Autodesk Inventor part; units mm, degrees
ref_plane "YZ Plane" through (0, 0, 0) normal (1, 0, 0) x (0, 1, 0)
ref_plane "XZ Plane" through (0, 0, 0) normal (0, 1, 0) x (-1, 0, 0)
ref_plane "XY Plane" through (0, 0, 0) normal (0, 0, 1) x (1, 0, 0)
sketch "Sketch1" plane through (0, 0, 0) normal (0, 0, 1) x (1, 0, 0)
  line L0 (2, 0) -> (8, 0)
  line L1 (10, 2) -> (10, 13)
  line L2 (8, 15) -> (2, 15)
  line L3 (0, 13) -> (0, 2)
  circle A0 centre (5, 7.5) radius 2.4
  arc A1 (10, 13) -> (8, 15) centre (8, 13) ccw
  arc A2 (2, 15) -> (0, 13) centre (2, 13) ccw
  arc A3 (0, 2) -> (2, 0) centre (2, 2) ccw
  arc A4 (8, 0) -> (10, 2) centre (8, 2) ccw
  point P0 (0, 0)
  point P1 (10, 15)
  point P2 (10, 0)
  point P3 (0, 15)
  dimension "d0" = 10
  dimension "d1" = 15
  dimension "d2" = 4.8
  dimension "d3" = 2
extrude "Extrusion1" add sketch "Sketch1" along normal blind 1.5
sketch "Sketch2" plane through (0, 0, 1.5) normal (0, 0, 1) x (1, 0, 0)
  circle A0 centre (5, 7.5) radius 2.4
  circle A1 centre (5, 7.5) radius 3.25
  point P0 (0, 0)
  dimension "d6" = 6.5
extrude "Extrusion2" add sketch "Sketch2" along normal blind 1
fillet "Fillet1" radius 0.5 1 edges at (1.75, 7.5, 1.5)
thread "Thread1"
fillet "Fillet2" radius 0.5 8 edges at (0.5858, 0.5858, 1.5) (5, 0, 1.5) (9.4142, 0.5858, 1.5) (10, 7.5, 1.5) (9.4142, 14.4142, 1.5) (5, 15, 1.5) (0.5858, 14.4142, 1.5) (0, 7.5, 1.5)
properties part number "M5 Tee Nut"
Work out the finished part from the listing and answer in its coordinate system (mm). A direction names the side the tool comes from. Round coordinates to 2 decimals unless told otherwise and drop trailing zeros. Write each loop counter-clockwise with the first axis right and the second up, starting at its lowest first coordinate (ties: lowest second). Pieces come first, ordered by that corner, then holes. Notation, with made-up numbers: M 56,33 L 61,33 A25 cw 61,63 Z; hole C 43,82 d8. An arc over 180 degrees is marked long. Use a Markdown table: item, result.
1) The part is cut by section B-B on x = 5. Give the vertices of the cut face in (y, z), plus the area to 3 significant figures.
Taken from the geometry:
| item | result |
|---|---|
| outline | M 0,0 L 5.1,0 L 5.1,2.5 L 4.25,2.5 L 4.25,2 A0.5 cw 3.75,1.5 L 0.5,1.5 A0.5 ccw 0,1 Z; M 9.9,0 L 15,0 L 15,1 A0.5 ccw 14.5,1.5 L 11.25,1.5 A0.5 cw 10.75,2 L 10.75,2.5 L 9.9,2.5 Z |
| area | 17.0 mm2 |
2) The part is cut by section A-A on y = 7.5. Give the vertices of the cut face in (x, z).
Taken from the geometry:
| item | result |
|---|---|
| outline | M 0,0 L 2.6,0 L 2.6,2.5 L 1.75,2.5 L 1.75,2 A0.5 cw 1.25,1.5 L 0.5,1.5 A0.5 ccw 0,1 Z; M 7.4,0 L 10,0 L 10,1 A0.5 ccw 9.5,1.5 L 8.75,1.5 A0.5 cw 8.25,2 L 8.25,2.5 L 7.4,2.5 Z |
3) Consider line 1 (Y direction, x = 5, z = 0.85); line 2 (Z direction, x = 7.25, y = 1.5); line 3 (X direction, y = 8.75, z = 0.85). Determine where each line is inside the solid, lowest interval first. Write a range as [from, to].
Taken from the geometry:
| item | result |
|---|---|
| line 1 | y = [0, 5.1], [9.9, 15] |
| line 2 | z = [0, 1.5] |
| line 3 | x = [0, 2.95], [7.05, 10] |
4) Which of the six approach directions +Z, -Z, +X, -X, +Y, -Y give full straight-line access (tool end or side, diameter ignored) to faces 5 (the face through (4, 5, 2.5)), 6 (the face through (3, 11, 1.5))?
Taken from the geometry:
| item | result |
|---|---|
| face 5 | +Z, +X, -X, +Y, -Y |
| face 6 | +Z |
5) The part is cut by section C-C on z = 1.3. Give the vertices of the cut face in (x, y), plus the area to 3 significant figures.
Taken from the geometry:
| item | result |
|---|---|
| outline | M 0.1,2 A1.9 ccw 2,0.1 L 8,0.1 A1.9 ccw 9.9,2 L 9.9,13 A1.9 ccw 8,14.9 L 2,14.9 A1.9 ccw 0.1,13 Z; hole C 5,7.5 d4.8 |
| area | 124 mm2 |
6) The part is cut by section D-D on z = 0.3. Give the vertices of the cut face in (x, y), plus the area to 3 significant figures.
Taken from the geometry:
| item | result |
|---|---|
| outline | M 0,2 A2 ccw 2,0 L 8,0 A2 ccw 10,2 L 10,13 A2 ccw 8,15 L 2,15 A2 ccw 0,13 Z; hole C 5,7.5 d4.8 |
| area | 128 mm2 |
7) Determine the mould class of faces 1 (the face through (6.75, 4.76, 2.25)), 2 (the face through (7.217, 8.419, 1.232)), 3 (the face through (7.2, 5.9, 0)), 4 (the face through (0.57, 14.4, 0.49)) for opening direction X: pulls with the +X half, pulls with the -X half, needs draft (parallel to the pull), parting line crosses it, or undercut.
Taken from the geometry:
| item | result |
|---|---|
| face 1 | parting line crosses it |
| face 2 | undercut |
| face 3 | needs draft |
| face 4 | pulls with the -X half |
8) A flat-ended cylindrical pin translates along its axis: pin 1 (1.5 mm diameter, centred on x = 1, z = 1.5, fed in from +Y). Find the tip coordinate at first contact, or state that the pin passes through.
Taken from the geometry:
| item | result |
|---|---|
| pin 1 | stops at y = 14.96 |
